```python
from build123d import *

# Parameters (mm, degrees)
F1_DEPTH = 20
F2_W     = 2
F2_H     = 18.9999999525
F2_W_2   = 8
F2_H_2   = 2
F2_H_3   = 19.0000000475
F3_DEPTH = 10
F4_R     = 1.5


with BuildPart() as f1:
    # F0 (on Top) → F1 (new body, symmetric)
    with BuildSketch(Plane.XY):
        Polygon((0, -1.5), (0, 0), (65, 0), (65, 2), (-3, 2), (-3, -3), (10, -3), (6.3068126328, -1.5), align=None)
    extrude(amount=F1_DEPTH, both=True)

    # F2 (on face) → F3 (join)
    with BuildSketch(Plane.YZ.offset(65)):
        with Locations((1, -10.5000000237)):
            Rectangle(F2_W, F2_H)
        with Locations((-4, -4.75e-08)):
            Rectangle(F2_W_2, F2_H_2)
        with Locations((1, -4.75e-08)):
            Rectangle(F2_W, F2_H_2)
        with Locations((6, -4.75e-08)):
            Rectangle(F2_W_2, F2_H_2)
        with Locations((1, 10.4999999763)):
            Rectangle(F2_W, F2_H_3)
    extrude(amount=F3_DEPTH)

    # F4
    f4_edges = [f1.edges().sort_by_distance(p)[0] for p in [
        (-3, -3, 0),
        (-3, 2, 0),
    ]]
    fillet(f4_edges, radius=F4_R)


solid = f1.part
```
Check sheet for the modelled part. Datum: model origin and axes. Units: mm. A direction names the side the tool comes from. Round coordinates to 2 decimals unless told otherwise and drop trailing zeros. Loops run counter-clockwise (first coordinate to the right, second up) from the corner with the lowest first, then second, coordinate; pieces in that order, holes last. Notation, with made-up numbers: (68.5, 48.25) - (124.5, 48.25) arc R37 ccw to (124.5, 86.25) - close; hole circle Ø11 at (19.25, 58). An arc over 180 degrees is marked (long way). Answer as a JSON object with one key per item and string values. Group by question number.
Q1. Sectioned sample at B-B, the plane z = 7.5. Enter the section's corners in (x, y), plus the area to 3 significant figures.
Q2. Mould release check, pull along Y, two halves, no side actions. Record for faces 1 (the face through (3, -1.5, 0)), 2 (the face through (35, 1, 20)), 3 (the face through (4, -3, 0)): released by +Y, released by -Y, zero draft, split by the parting line, or undercut.
Q3. Sectioned sample at D-D, the plane x = 55.5. Enter the section's corners in (y, z).
Q4. Gauge pin test, flat ends, axial feed: P1, Ø0.6, axis at y = -6, z = 0.5, coming from the -X side; P2, Ø12, axis at x = 50, z = -9, coming from the -Y side; P3, Ø20, axis at x = 35, z = 5, coming from the +Y side. Record the tip position at first contact, or that the pin passes through.
Q5. Scan lines: line 1 along Y through (x, z) = (5, -14); line 2 along Y through (x, z) = (29.5, 3); line 3 along X through (y, z) = (-1.25, 18.5). Record each from-to range of solid material in increasing order. Write a range as [from, to].
Q6. Sectioned sample at A-A, the plane x = 70. Enter the section's corners in (y, z).
Q7. Sectioned sample at C-C, the plane y = 8.5. Enter the section's corners in (x, z).
Q8. Set-up check for faces 4 (the face through (70, 6, -1)), 5 (the face through (65, 6, 0)), 6 (the face through (70, -4, 1)), 7 (the face through (70, 6, 1)), 8 (the face through (70, -4, -1)): record each of +Z, -Z, +X, -X, +Y, -Y from which the full face is reachable in a straight line by a thin tool's end or side.
Solution:
{
 "1": {"outline": "(-3, -1.5) arc R1.5 ccw to (-1.5, -3) - (10, -3) - (6.31, -1.5) - (0, -1.5) - (0, 0) - (75, 0) - (75, 2) - (-1.5, 2) arc R1.5 ccw to (-3, 0.5) - close", "area": "176 mm²"},
 "2": {"face 1": "undercut", "face 2": "zero draft", "face 3": "released by -Y"},
 "3": {"outline": "(0, -20) - (2, -20) - (2, 20) - (0, 20) - close"},
 "4": {"P1": "stops at x = 65", "P2": "stops at y = 0", "P3": "stops at y = 2"},
 "5": {"line 1": "y = [-3, -1.5], [0, 2]", "line 2": "y = [0, 2]", "line 3": "x = [-3, 0]"},
 "6": {"outline": "(-8, -1) - (0, -1) - (0, -20) - (2, -20) - (2, -1) - (10, -1) - (10, 1) - (2, 1) - (2, 20) - (0, 20) - (0, 1) - (-8, 1) - close"},
 "7": {"outline": "(65, -1) - (75, -1) - (75, 1) - (65, 1) - close"},
 "8": {"face 4": "-Z, +X, -X, +Y", "face 5": "+Z, -Z, -X, +Y", "face 6": "+Z, +X, -Y", "face 7": "+Z, +X, -X, +Y", "face 8": "-Z, +X, -Y"}
}
